```python
from build123d import *

# Parameters (mm, degrees)
BOSS_EXTRUDE3_DEPTH      = 10
BOSS_EXTRUDE5_DEPTH      = 2
BOSS_EXTRUDE5_DEPTH_BACK = 2
SKETCH4_R                = 1.6
CUT_EXTRUDE1_DEPTH       = 11
SKETCH5_R                = 1
CUT_EXTRUDE3_DEPTH       = 8


with BuildPart() as part:
    # Sketch2 → Boss-Extrude3 (new body)
    with BuildSketch(Plane(origin=(0, 0, 0), x_dir=(1, 0, 0), z_dir=(0, 1, 0))):
        with BuildLine():
            Line((0, -1.6), (-9.871170143, -1.6))
            ThreePointArc((-9.871170143, -1.6), (-10, 0), (-9.871170143, 1.6))
            Line((-9.871170143, 1.6), (0, 1.6))
            ThreePointArc((0, 1.6), (1.6, 0), (0, -1.6))
        make_face()
    extrude(amount=BOSS_EXTRUDE3_DEPTH)

    # Sketch3 → Boss-Extrude5 (add, two sides)
    with BuildSketch(Plane(origin=(0, 5, 0), x_dir=(1, 0, 0), z_dir=(0, 1, 0))) as boss_extrude5_sk:
        with BuildLine():
            Line((3, -4), (-9.16515139, -4))
            ThreePointArc((-9.16515139, -4), (-10, 0), (-9.16515139, 4))
            Line((-9.16515139, 4), (3, 4))
            ThreePointArc((3, 4), (7, 0), (3, -4))
        make_face()
    extrude(amount=BOSS_EXTRUDE5_DEPTH)
    extrude(boss_extrude5_sk.sketch, amount=-BOSS_EXTRUDE5_DEPTH_BACK)

    # Sketch4 → Cut-Extrude1 (cut, through all)
    with BuildSketch(Plane(origin=(0, 10, 0), x_dir=(1, 0, 0), z_dir=(0, 1, 0))):
        Circle(SKETCH4_R)
    extrude(amount=-CUT_EXTRUDE1_DEPTH, mode=Mode.SUBTRACT)

    # Sketch5 → Cut-Extrude3 (cut, through all)
    with BuildSketch(Plane(origin=(0, 7, 0), x_dir=(1, 0, 0), z_dir=(0, 1, 0))):
        with Locations((4, 0)):
            Circle(SKETCH5_R)
    extrude(amount=-CUT_EXTRUDE3_DEPTH, mode=Mode.SUBTRACT)


solid = part.part
```
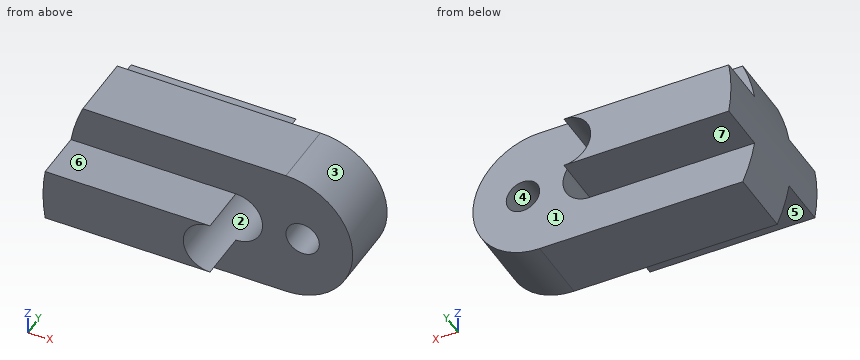
Verification items for the finished model (mm, model axes). Face numbers are marked on the shaded views. A direction names the side the tool comes from. Give positions to 0.01 mm unless a question says otherwise; leave off trailing zeros. Write each loop counter-clockwise with the first axis right and the second up, starting at its lowest first coordinate (ties: lowest second). Pieces come first, ordered by that corner, then holes. Notation, with made-up numbers: (-23, -22) - (-7, -22) arc R23 ccw to (-7, -3) - close; hole circle Ø2 at (78.5, 25.25). An arc over 180 degrees is marked (long way). Put each result on its own line as item: value.
Q1. Scan lines: probe 1 along X at (y, z) = (5.75, 0); probe 2 along Z at (x, y) = (-1.25, 2); probe 3 along Z at (x, y) = (0.25, 4.5). Record each from-to range of solid material in increasing order. Write a range as from..to.
Result:
probe 1: -10..-1.6, 1.6..3, 5..7
probe 2: -1.6..-1, 1..1.6
probe 3: -4..-1.58, 1.58..4
Q2. Section check D-D on x = 4. Record the cut outline in (y, z).
Result:
outline: (3, -3.87) - (7, -3.87) - (7, -1) - (3, -1) - close; (3, 1) - (7, 1) - (7, 3.87) - (3, 3.87) - close
Q3. Mould release check, pull along Z, two halves, no side actions. Record for the marked faces 1, 2, 3 and 4: released by +Z, released by -Z, zero draft, split by the parting line, or undercut.
Result:
face 1: zero draft
face 2: undercut
face 3: split by the parting line
face 4: undercut
Q4. Section check B-B on x = -2. Record the cut outline in (y, z).
Result:
outline: (0, -1.6) - (3, -1.6) - (3, -4) - (7, -4) - (7, -1.6) - (10, -1.6) - (10, 1.6) - (7, 1.6) - (7, 4) - (3, 4) - (3, 1.6) - (0, 1.6) - close
Q5. Set-up check for the marked faces 5, 6 and 7: record each of +Z, -Z, +X, -X, +Y, -Y from which the full face is reachable in a straight line by a thin tool's end or side.
Result:
face 5: -Z, +X, -X, -Y
face 6: +Z, +X, -X, -Y
face 7: -Z, +X, -X, +Y
Q6. Section check A-A on z = 0. Record the cut outline in (x, y), and give its area (3 significant figures).
Result:
outline: (-10, 0) - (-1.6, 0) - (-1.6, 10) - (-10, 10) - close; (1.6, 3) - (3, 3) - (3, 7) - (1.6, 7) - close; (5, 3) - (7, 3) - (7, 7) - (5, 7) - close
area: 97.6 mm2
Q7. Section check C-C on y = 6. Record the cut outline in (x, z).
Result:
outline: (-9.17, -4) - (3, -4) arc R4 ccw to (3, 4) - (-9.17, 4) arc R10 ccw to start; hole circle Ø3.2 at (0, 0); hole circle Ø2 at (4, 0)
Q8. Depth check by flat-ended pin: P1, Ø1, axis at x = -8, y = 8.5, coming from the +Z side; P2, Ø0.9, axis at x = -4.5, y = 2, coming from the -Z side; P3, Ø3, axis at x = 0, z = 0, coming from the +Y side (3 decimals). Enter the tip coordinate at first touch or a pass-through.
Result:
P1: z = 1.6
P2: z = -1.6
P3: through
